Design review of the part built by this model. Coordinates are the model's own, in mm. A direction names the side the tool comes from. Coordinates: 2 decimals unless noted, no trailing zeros. Loops run counter-clockwise (first coordinate to the right, second up) from the corner with the lowest first, then second, coordinate; pieces in that order, holes last. Notation, with made-up numbers: (43.5, 7) -> (80.5, 7) arc R19 cw to (80.5, 25) -> close; hole circle Ø8 at (-32, 84.5). An arc over 180 degrees is marked (long way). Use one line per item in the form item = value. Start each with the question number.
1. Consider section A-A (y = 0). State the section outline as (x, z) points, then the cut area to 3 significant figures.
2. For pin 1 (1.1 mm diameter, centred on y = -0.5, z = -8, fed in from -X); pin 2 (2 mm diameter, centred on y = -1.5, z = -2, fed in from +X); pin 3 (3.5 mm diameter, centred on x = 28.75, y = 0, fed in from +Z), all flat-tipped, find the tip position at first contact; note any pin that passes through.
3. Consider section B-B (x = 37.5). State the section outline as (y, z) points, then the cut area to 3 significant figures.
4. Consider section D-D (x = 28.75). State the section outline as (y, z) points.
5. Consider section C-C (y = 3). State the section outline as (x, z) points, then the cut area to 3 significant figures.
6. Machinability: for faces 4 (the face through (32, 0, -8)), 5 (the face through (31.67, -0.04, -3.21)), 6 (the face through (34, -3.5, -6)), which of the approach directions +Z, -Z, +X, -X, +Y, -Y give a long, thin tool a straight path to every point of the face, cutting with its end or side? Answer none if there is none.
7. The part is to be moulded in two halves that separate along Z. For faces 1 (the face through (30, 1, -9.1)), 2 (the face through (34, 3.5, -6)), 3 (the face through (41.6, 0.05, -1.97)), say which applies: released by +Z, released by -Z, zero draft, split by the parting line, or undercut.
8. Wall thickness on line 1 (Y direction, x = 28.75, z = -9.4); line 2 (Y direction, x = 29.5, z = -2.25); line 3 (Z direction, x = 37.5, y = 1): over which ranges is each line inside the solid? List them lowest first. Write a range as from..to.
from build123d import *

# Parameters (mm, degrees)
CYLINDER241_R      = 2.8
CYLINDER241_DEPTH  = 10
BOX164_W           = 7
BOX164_H           = 10
BOX164_DEPTH       = 3
BOX161_W           = 10
BOX161_H           = 10
BOX161_DEPTH       = 2.2
BOX160_W           = 10
BOX160_H           = 5.5
BOX160_DEPTH       = 18
CHAMFER023_1_SIZE2 = 4
CHAMFER023_1_SIZE  = 17
CHAMFER023_2_SIZE2 = 0.8
CHAMFER023_2_SIZE  = 17
CYLINDER238_R      = 1.4
CYLINDER238_DEPTH  = 19
CYLINDER239_R      = 2
CYLINDER239_DEPTH  = 10
BOX159_W           = 18
BOX159_H           = 7
BOX159_DEPTH       = 10
FILLET097_R        = 4.9


with BuildPart() as zylinder243:
    # Cylinder241 → Cylinder241 (new body)
    with BuildSketch(Plane(origin=(28.5, 0, -16.5), x_dir=(1, 0, 0), z_dir=(0, 0, 1))):
        Circle(CYLINDER241_R)
    extrude(amount=CYLINDER241_DEPTH)


with BuildPart() as cut111:
    # Box164 → Box164 (new body)
    with BuildSketch(Plane(origin=(21, -5, -12), x_dir=(1, 0, 0), z_dir=(0, 0, 1))):
        with Locations((3.5, 5)):
            Rectangle(BOX164_W, BOX164_H)
    extrude(amount=BOX164_DEPTH)

    # Cut111: cut Zylinder243
    add(zylinder243.part, mode=Mode.SUBTRACT)


with BuildPart() as obj1:
    # Box161 → Box161 (new body)
    with BuildSketch(Plane(origin=(22, -5, -9.1), x_dir=(1, 0, 0), z_dir=(0, 0, 1))):
        with Locations((5, 5)):
            Rectangle(BOX161_W, BOX161_H)
    extrude(amount=BOX161_DEPTH)


with BuildPart() as chamfer023:
    # Box160 → Box160 (new body)
    with BuildSketch(Plane(origin=(21.8, -2.75, -7), x_dir=(1, 0, 0), z_dir=(0, 0, 1))):
        with Locations((5, 2.75)):
            Rectangle(BOX160_W, BOX160_H)
    extrude(amount=BOX160_DEPTH)

    # Chamfer023 1
    chamfer023_1_edges = [chamfer023.edges().sort_by_distance(p)[0] for p in [
        (21.8, 0, 11),
    ]]
    chamfer023_1_side = chamfer023.faces().sort_by_distance((21.8, 0, 2))[0]
    chamfer(chamfer023_1_edges, length=CHAMFER023_1_SIZE, length2=CHAMFER023_1_SIZE2, reference=chamfer023_1_side)

    # Chamfer023 2
    chamfer023_2_edges = [chamfer023.edges().sort_by_distance(p)[0] for p in [
        (31.8, 0, 11),
    ]]
    chamfer023_2_side = chamfer023.faces().sort_by_distance((31.8, 0, 2))[0]
    chamfer(chamfer023_2_edges, length=CHAMFER023_2_SIZE, length2=CHAMFER023_2_SIZE2, reference=chamfer023_2_side)


with BuildPart() as fusion158:
    # Cylinder238 → Cylinder238 (new body)
    with BuildSketch(Plane(origin=(28.75, 0, -11.5), x_dir=(1, 0, 0), z_dir=(0, 0, 1))):
        Circle(CYLINDER238_R)
    extrude(amount=CYLINDER238_DEPTH)

    # Fusion158: union obj1, Chamfer023
    add(obj1.part)
    add(chamfer023.part)


with BuildPart() as fusion159:
    # Cylinder239 → Cylinder239 (new body)
    with BuildSketch(Plane(origin=(37.5, 5, -5.5), x_dir=(1, 0, 0), z_dir=(0, -1, 0))):
        Circle(CYLINDER239_R)
    extrude(amount=CYLINDER239_DEPTH)

    # Fusion159: union Fusion158
    add(fusion158.part)


with BuildPart() as cut112:
    # Box159 → Box159 (new body)
    with BuildSketch(Plane(origin=(25, -3.5, -10.5), x_dir=(1, 0, 0), z_dir=(0, 0, 1))):
        with Locations((9, 3.5)):
            Rectangle(BOX159_W, BOX159_H)
    extrude(amount=BOX159_DEPTH)

    # Fillet097
    fillet097_edges = [cut112.edges().sort_by_distance(p)[0] for p in [
        (43, 0, -0.5),
        (43, 0, -10.5),
    ]]
    fillet(fillet097_edges, radius=FILLET097_R)

    # Cut109: cut Fusion159
    add(fusion159.part, mode=Mode.SUBTRACT)

    # Cut112: cut Cut111
    add(cut111.part, mode=Mode.SUBTRACT)


solid = cut112.part
Geometry check:
q1.outline = (25.7, -10.5) -> (27.35, -10.5) -> (27.35, -9.1) -> (25.7, -9.1) -> close; (30.15, -10.5) -> (38.1, -10.5) arc R4.9 ccw to (43, -5.6) -> (43, -5.4) arc R4.9 ccw to (38.1, -0.5) -> (31.54, -0.5) -> (31.8, -6) -> (31.8, -6.9) -> (32, -6.9) -> (32, -9.1) -> (30.15, -9.1) -> close; hole circle Ø4 at (37.5, -5.5)
q1.area = 94.0 mm²
q2.pin_1 = 32
q2.pin_2 = 42.37
q2.pin_3 = -9.1
q3.outline = (-3.5, -10.5) -> (3.5, -10.5) -> (3.5, -7.5) -> (-3.5, -7.5) -> close; (-3.5, -3.5) -> (3.5, -3.5) -> (3.5, -0.5) -> (-3.5, -0.5) -> close
q3.area = 42.0 mm²
q4.outline = (-3.5, -10.5) -> (-1.4, -10.5) -> (-1.4, -9.1) -> (-3.5, -9.1) -> close; (-3.5, -6.9) -> (-2.75, -6.9) -> (-2.75, -0.5) -> (-3.5, -0.5) -> close; (1.4, -10.5) -> (3.5, -10.5) -> (3.5, -9.1) -> (1.4, -9.1) -> close; (2.75, -6.9) -> (3.5, -6.9) -> (3.5, -0.5) -> (2.75, -0.5) -> close
q5.outline = (25, -6.9) -> (32, -6.9) -> (32, -9.1) -> (28, -9.1) -> (28, -10.5) -> (38.1, -10.5) arc R4.9 ccw to (43, -5.6) -> (43, -5.4) arc R4.9 ccw to (38.1, -0.5) -> (25, -0.5) -> close; hole circle Ø4 at (37.5, -5.5)
q5.area = 138 mm²
q6.face_4 = -X, +Y, -Y
q6.face_5 = -X
q6.face_6 = +Z, -Z, +X, -X, -Y
q7.face_1 = undercut
q7.face_2 = zero draft
q7.face_3 = released by +Z
q8.line_1 = -3.5..-1.4, 1.4..3.5
q8.line_2 = -3.5..-2.75, 2.75..3.5
q8.line_3 = -10.5..-7.5, -3.5..-0.5
